from build123d import *

# Parameters (mm, degrees)
CHAMFER2_SIZE = 0.5953125


with BuildPart() as part:
    # Sketch3 → Revolve1 (revolve)
    with BuildSketch(Plane.XY, mode=Mode.PRIVATE) as revolve1_sk:
        with BuildLine():
            Line((-10.702925, 2.8702), (-10.702925, 4.708465665))
            Line((-10.702925, 4.708465665), (-5.794375, 4.7625))
            Line((-5.794375, 4.7625), (-5.794375, 4.625018467))
            Line((-5.794375, 4.625018467), (-5.55625, 4.493023624))
            Line((-5.55625, 4.493023624), (-5.55625, 4.42689468))
            ThreePointArc((-5.55625, 4.42689468), (-5.538212237, 4.384141282), (-5.495001316, 4.367228853))
            Line((-5.495001316, 4.367228853), (-4.549371052, 4.391991053))
            ThreePointArc((-4.549371052, 4.391991053), (-4.419738289, 4.341253768), (-4.365625, 4.212993574))
            Line((-4.365625, 4.212993574), (-4.365625, 1.575604266))
            Line((-4.365625, 1.575604266), (-5.622925, 1.575604266))
            Line((-5.622925, 1.575604266), (-5.622925, 2.8702))
            Line((-5.622925, 2.8702), (-10.702925, 2.8702))
        make_face()
    revolve(revolve1_sk.sketch.rotate(Axis((-9.128125, 0, 0), (1, 0, 0)), 180), axis=Axis((-9.128125, 0, 0), (1, 0, 0)))

    # Sketch4 → Revolve2 (revolve)
    with BuildSketch(Plane.XY, mode=Mode.PRIVATE) as revolve2_sk:
        Polygon((-10.702925, 2.8702), (-5.622925, 2.8702), (-5.622925, 1.7526), (9.128125, 1.7526), (9.128125, 0), (-10.702925, 0), align=None)
    revolve(revolve2_sk.sketch.rotate(Axis((-10.702925, 0, 0), (1, 0, 0)), 180), axis=Axis((-10.702925, 0, 0), (1, 0, 0)))

    # Chamfer2
    chamfer2_edges = [part.edges().sort_by_distance(p)[0] for p in [
        (9.128125, 1.7526, 0),
    ]]
    chamfer(chamfer2_edges, length=CHAMFER2_SIZE)


solid = part.part
Can you work these out from the model? Positions are in its coordinate system, mm. A direction names the side the tool comes from. Give positions to 0.01 mm unless a question says otherwise; leave off trailing zeros. Loops run counter-clockwise (first coordinate to the right, second up) from the corner with the lowest first, then second, coordinate; pieces in that order, holes last. Notation, with made-up numbers: (76.5, 76.5) -> (126.5, 76.5) arc R19 ccw to (126.5, 105.5) -> close; hole circle Ø10 at (15, 19). An arc over 180 degrees is marked (long way). Return JSON: item names as keys, results as strings.
Q1. I need wall thicknesses on probe 1 along X at (y, z) = (-2.25, -1.5); probe 2 along Y at (x, z) = (3.5, 0.5); probe 3 along Z at (x, y) = (2.25, 1). Which ranges of each line are inside material? Lowest first, please.
Checks:
{"probe 1": "x = -10.7 to -4.37", "probe 2": "y = -1.68 to 1.68", "probe 3": "z = -1.44 to 1.44"}
Q2. On a 3-axis mill with a long thin cutter (end or side, diameter ignored), from which of +Z, -Z, +X, -X, +Y, -Y can I reach the whole of each face in a straight line? I mean faces 5 (the face through (-10.703, 0, 0)), 6 (the face through (-4.366, -2, 0)). Say none if no direction works.
Checks:
{"face 5": "+Z, -Z, -X, +Y, -Y", "face 6": "+X"}
Q3. I want a section at B-B, the plane x = -7.75. List the corners of the cut face in (y, z) for me, then the cut area to 3 significant figures.
Checks:
{"outline": "circle Ø9.48 at (0, 0)", "area": "70.6 mm2"}
Q4. I want a section at A-A, the plane x = -0.75. List the corners of the cut face in (y, z) for me.
Checks:
{"outline": "circle Ø3.51 at (0, 0)"}
Q5. We'd pull the mould along X, two halves only. Please class faces 1 (the face through (2.17, -1.67, -0.53)), 2 (the face through (-8.214, 0.617, -4.696)), 3 (the face through (-5.121, -4.175, -1.315)), 4 (the face through (9.128, 0, 0)): released by +X, released by -X, zero draft, split by the parting line, or undercut.
Checks:
{"face 1": "zero draft", "face 2": "released by -X", "face 3": "undercut", "face 4": "released by +X"}
Q6. For pin 1 Ø2 at (y, z) = (-2.5, -3.5) entering from +X; pin 2 Ø1 at (x, y) = (0, -0.5) entering from +Z; pin 3 Ø5 at (x, z) = (2, 0.5) entering from +Y, each with a flat end and sliding along its axis, tell me the tip position at first contact or that it passes through.
Checks:
{"pin 1": "stops at x = -4.37", "pin 2": "stops at z = 1.75", "pin 3": "stops at y = 1.75"}
